Here's the drawing with two shaded views (mm, measured from the low corner). I have some questions. A direction names the side the tool comes from. Round coordinates to 2 decimals unless told otherwise and drop trailing zeros. Order: outer loops, then holes, each group sorted by start corner. A loop starts at its lowest first (then second) coordinate and runs counter-clockwise, first axis right, second up. Notation, with made-up numbers: (-8, 8.5) - (25, 8.5) arc R16 cw to (25, 19.5) - close; hole circle Ø7 at (-17, -2.5). An arc over 180 degrees is marked (long way). Return JSON: item names as keys, results as strings. Group by question number.
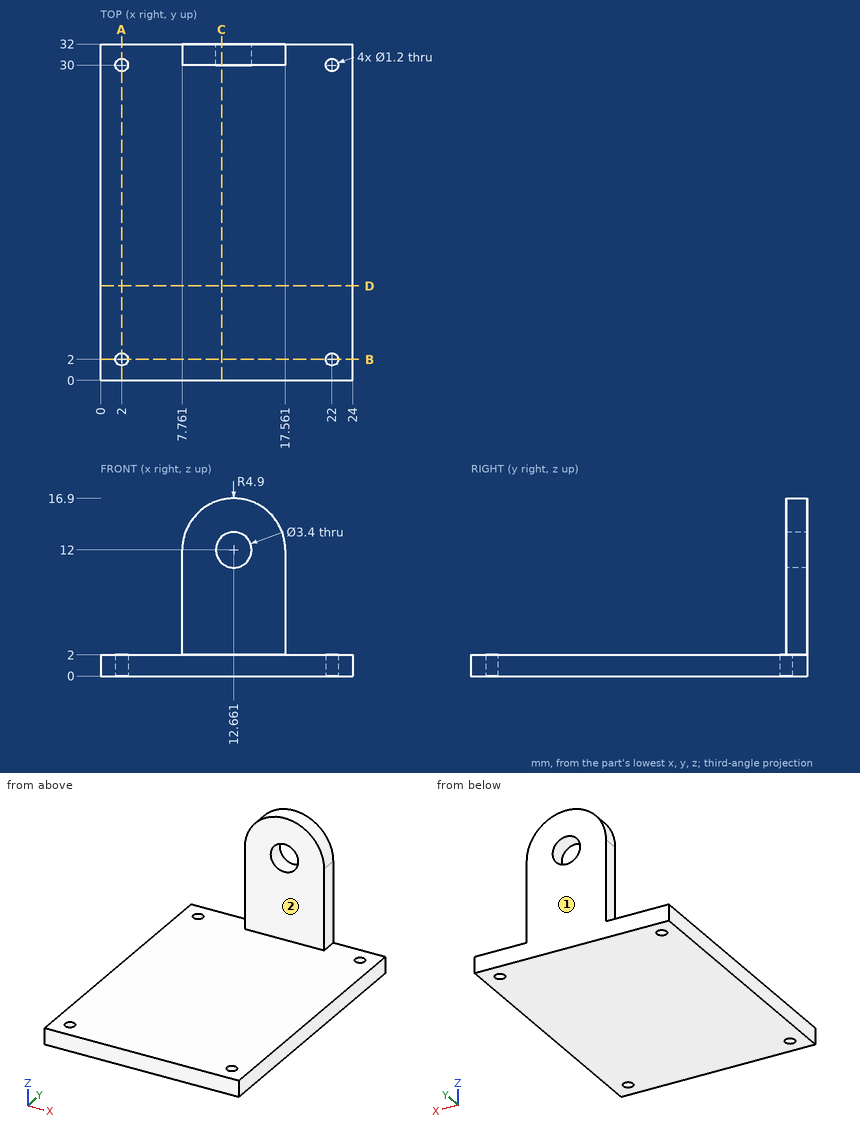
1) I want a section at C-C, the plane x = 11.5. List the corners of the cut face in (y, z) for me.
2) I want a section at D-D, the plane y = 9. List the corners of the cut face in (x, z) for me.
3) Will these pins go through, and if not, where does the flat tip stop? pin 1 (3 mm diameter, centred on x = 14, y = 16, fed in from +Z); pin 2 (1.6 mm diameter, centred on y = 31, z = 7.5, fed in from +X); pin 3 (1.6 mm diameter, centred on y = 31.5, z = 7.5, fed in from -X).
4) I want a section at A-A, the plane x = 2. List the corners of the cut face in (y, z) for me.
5) I want a section at B-B, the plane y = 2. List the corners of the cut face in (x, z) for me.
6) For the marked faces 1 and 2, which set-ups out of +Z, -Z, +X, -X, +Y, -Y let a thin tool reach every point of the face, with its end or its side?
7) If I drill on line 1 along X through (y, z) = (2, 0.6); line 2 along Z through (x, y) = (8.25, 9); line 3 along Y through (x, z) = (10.5, 2.25), over which ranges is the centre line in solid material (lowest first)? Write a range as from..to.
Outcome:
{
 "1": {"outline": "(0, 0) - (32, 0) - (32, 10.76) - (30, 10.76) - (30, 2) - (0, 2) - close; (30, 13.24) - (32, 13.24) - (32, 16.76) - (30, 16.76) - close"},
 "2": {"outline": "(0, 0) - (24, 0) - (24, 2) - (0, 2) - close"},
 "3": {"pin 1": "z = 2", "pin 2": "x = 17.56", "pin 3": "x = 7.76"},
 "4": {"outline": "(0, 0) - (1.4, 0) - (1.4, 2) - (0, 2) - close; (2.6, 0) - (29.4, 0) - (29.4, 2) - (2.6, 2) - close; (30.6, 0) - (32, 0) - (32, 2) - (30.6, 2) - close"},
 "5": {"outline": "(0, 0) - (1.4, 0) - (1.4, 2) - (0, 2) - close; (2.6, 0) - (21.4, 0) - (21.4, 2) - (2.6, 2) - close; (22.6, 0) - (24, 0) - (24, 2) - (22.6, 2) - close"},
 "6": {"face 1": "+Z, -Z, +X, -X, +Y", "face 2": "+Z, +X, -X, -Y"},
 "7": {"line 1": "0..1.4, 2.6..21.4, 22.6..24", "line 2": "0..2", "line 3": "30..32"}
}
